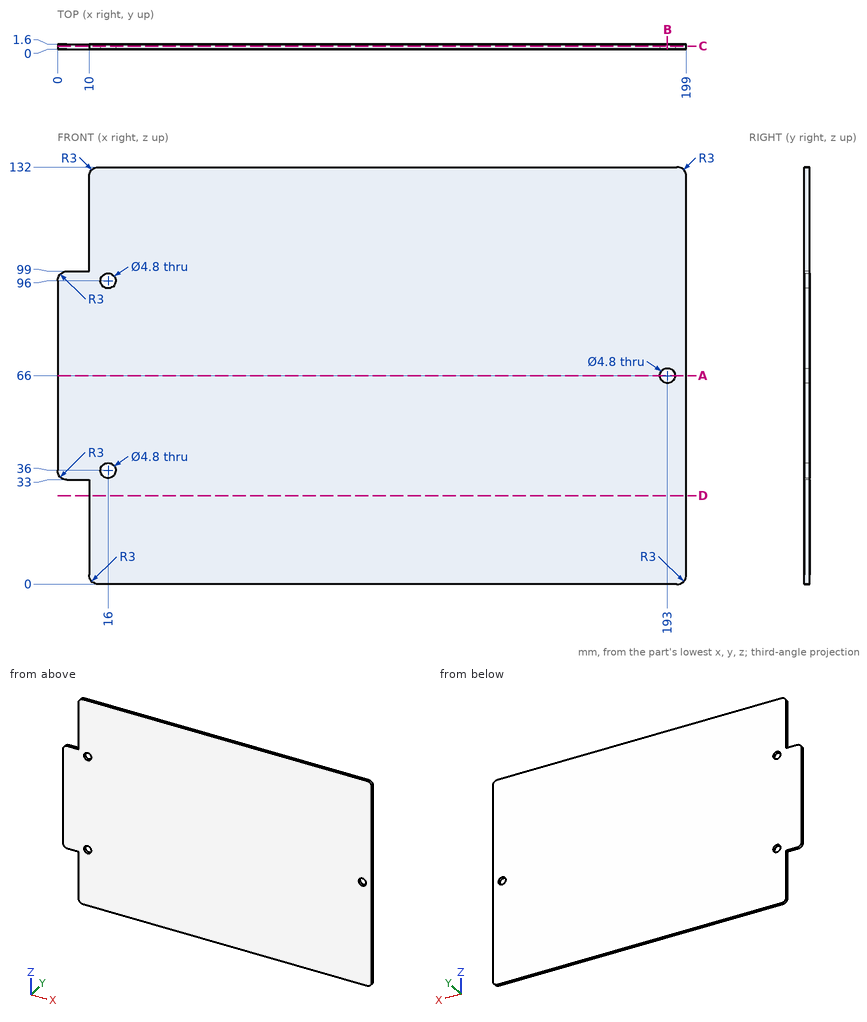
The drawing under review shows one solid part. Ordinate dimensions are in mm from its lowest x, y, z. Coordinates: 2 decimals unless noted, no trailing zeros. Write each loop counter-clockwise with the first axis right and the second up, starting at its lowest first coordinate (ties: lowest second). Pieces come first, ordered by that corner, then holes.
1) Add section D-D (z = 28). Write out the cut boundary in (x, y), plus the area to 3 significant figures.
2) Add section C-C (y = 0.95). Write out the cut boundary in (x, z).
3) Add section A-A (z = 66). Write out the cut boundary in (x, y).
4) Add section B-B (x = 193). Write out the cut boundary in (y, z).
5) To check wall thickness, follow L1, parallel to X at y = 1.05, z = 66; L2, parallel to X at y = 0.45, z = 96; L3, parallel to Z at x = 193, y = 0.8. State the ranges of each line that lie inside material, in increasing order.
6) Insertion check: pin 1 (0.5 mm diameter, centred on y = 0.5, z = 20.5, fed in from -X). The pin has a flat end and moves straight along its axis. Give the tip position at first contact, or say it passes through.
Check result:
1. outline: (10, 0) - (199, 0) - (199, 1.6) - (10, 1.6) - close
1. area: 302 mm2
2. outline: (0, 36) arc R3 ccw to (3, 33) - (10, 33) - (10, 3) arc R3 ccw to (13, 0) - (196, 0) arc R3 ccw to (199, 3) - (199, 129) arc R3 ccw to (196, 132) - (13, 132) arc R3 ccw to (10, 129) - (10, 99) - (3, 99) arc R3 ccw to (0, 96) - close; hole circle Ø4.8 at (16, 36); hole circle Ø4.8 at (16, 96); hole circle Ø4.8 at (193, 66)
3. outline: (0, 0) - (190.6, 0) - (190.6, 1.6) - (0, 1.6) - close; (195.4, 0) - (199, 0) - (199, 1.6) - (195.4, 1.6) - close
4. outline: (0, 0) - (1.6, 0) - (1.6, 63.6) - (0, 63.6) - close; (0, 68.4) - (1.6, 68.4) - (1.6, 132) - (0, 132) - close
5. L1: x = 0 to 190.6, 195.4 to 199
5. L2: x = 0 to 13.6, 18.4 to 199
5. L3: z = 0 to 63.6, 68.4 to 132
6. pin 1: stops at x = 10
